from build123d import *

# Parameters (mm, degrees)
SKETCH1_W           = 2400
SKETCH1_H           = 225
BOSS_EXTRUDE1_DEPTH = 10
BOSS_EXTRUDE2_START = 40
BOSS_EXTRUDE2_DEPTH = 70
BOSS_EXTRUDE5_DEPTH = 110
BOSS_EXTRUDE6_DEPTH = 105


with BuildPart() as part:
    # Sketch1 → Boss-Extrude1 (new body)
    with BuildSketch(Plane(origin=(0, 0, 0), x_dir=(1, 0, 0), z_dir=(0, 1, 0))):
        Rectangle(SKETCH1_W, SKETCH1_H)
    extrude(amount=BOSS_EXTRUDE1_DEPTH)

    # Sketch4 → Boss-Extrude2 (add)
    with BuildSketch(Plane.XY.offset(BOSS_EXTRUDE2_START)):
        Polygon((600, 10), (425, 10), (448.609614239, 40), (573.609614239, 40), align=None)
    extrude(amount=BOSS_EXTRUDE2_DEPTH)

    # Sketch10 → Boss-Extrude5 (add)
    with BuildSketch(Plane.XY):
        Polygon((-75, 10), (100, 10), (73.609614239, 40), (-51.390385761, 40), align=None)
    extrude(amount=-BOSS_EXTRUDE5_DEPTH)

    # Sketch11 → Boss-Extrude6 (add, symmetric)
    with BuildSketch(Plane.XY):
        Polygon((-575, 10), (-400, 10), (-426.390385761, 40), (-551.390385761, 40), align=None)
    extrude(amount=BOSS_EXTRUDE6_DEPTH, both=True)


solid = part.part
Model file for the job. Use its own axes, mm. Give positions to 0.01 mm unless a question says otherwise; leave off trailing zeros. Loops run counter-clockwise (first coordinate to the right, second up) from the corner with the lowest first, then second, coordinate; pieces in that order, holes last.
Item 1: Drop flat-ended pins along their axis: P1, Ø9, axis at x = 40.5, y = 25.5, coming from the +Z side; P2, Ø9, axis at x = 497.5, y = 31, coming from the -Z side; P3, Ø10, axis at x = -116, z = 4, coming from the +Y side; P4, Ø8, axis at x = -146, z = -69, coming from the -Y side. Give the stop position or say it passes through.
Check values:
P1: stops at z = 0
P2: stops at z = 40
P3: stops at y = 10
P4: stops at y = 0
Item 2: Slice it at D-D (x = -900). Write the cut outline in (y, z).
Check values:
outline: (0, -112.5) - (10, -112.5) - (10, 112.5) - (0, 112.5) - close
Item 3: Slice it at C-C (x = 514). Write the cut outline in (y, z).
Check values:
outline: (0, -112.5) - (10, -112.5) - (10, 40) - (40, 40) - (40, 110) - (10, 110) - (10, 112.5) - (0, 112.5) - close
Item 4: Drill centre lines: line 1 along Z through (x, y) = (532, 38); line 2 along Y through (x, z) = (-843, 15); line 3 along X through (y, z) = (38.5, 42.5). Where is each one in solid material? Low to high.
Check values:
line 1: z = 40 to 110
line 2: y = 0 to 10
line 3: x = -552.57 to -425.07, 447.43 to 574.93
Item 5: Mould opens along X. For faces 1 (the face through (510, 40, 75)), 2 (the face through (-17, 10, 23)) say: +X half, -X half, draft (parallel to the pull), parting line (faces both ways), or undercut.
Check values:
face 1: draft
face 2: undercut
Item 6: Slice it at B-B (z = -41). Write the cut outline in (x, y).
Check values:
outline: (-1200, 0) - (1200, 0) - (1200, 10) - (100, 10) - (73.61, 40) - (-51.39, 40) - (-75, 10) - (-400, 10) - (-426.39, 40) - (-551.39, 40) - (-575, 10) - (-1200, 10) - close
Item 7: Slice it at A-A (y = 23). Write the cut outline in (x, z), plus the area to 3 significant figures.
Check values:
outline: (-564.77, -105) - (-411.44, -105) - (-411.44, 105) - (-564.77, 105) - close; (-64.77, -110) - (88.56, -110) - (88.56, 0) - (-64.77, 0) - close; (435.23, 40) - (588.56, 40) - (588.56, 110) - (435.23, 110) - close
area: 59,800 mm2
